from build123d import *

# Parameters (mm, degrees)
CROQUIS1_R              = 9.525
SALIENTE_EXTRUIR1_DEPTH = 10
CROQUIS2_R              = 9.525


with BuildPart() as part:
    # Croquis1 → Saliente-Extruir1 (new body)
    with BuildSketch(Plane(origin=(0, 0, 0), x_dir=(1, 0, 0), z_dir=(0, 1, 0))):
        with Locations(Location((0, 0, 0), (0, 0, 270))):
            Circle(CROQUIS1_R)
    extrude(amount=-SALIENTE_EXTRUIR1_DEPTH)

    # Barrer1: sweep along a curve in space
    with BuildLine() as barrer1_path:
        Line((0, -10, 0), (0, -50, 0))
        ThreePointArc((0, -50, 0), (4.393398282, -60.606601718, 0), (15, -65, 0))
        Line((15, -65, 0), (35, -65, 0))
        ThreePointArc((35, -65, 0), (45.606601718, -69.393398282, 0), (50, -80, 0))
        Line((50, -80, 0), (50, -145, 0))
        ThreePointArc((50, -145, 0), (54.393398282, -155.606601718, 0), (65, -160, 0))
        Line((65, -160, 0), (805, -160, 0))
        ThreePointArc((805, -160, 0), (815.606601718, -155.606601718, 0), (820, -145, 0))
        Line((820, -145, 0), (820, 175, 0))
        ThreePointArc((820, 175, 0), (820, 185.606601718, 4.393398282), (820, 190, 15))
        Line((820, 190, 15), (820, 190, 100))
    # Croquis2 → Barrer1 (sweep)
    with BuildSketch(Plane.XZ.offset(10)):
        Circle(CROQUIS2_R)
    sweep(path=barrer1_path.line)


solid = part.part
The listing builds one solid part. Answer for the finished solid, in the listing's coordinates (mm). A direction names the side the tool comes from. Give positions to 0.01 mm unless a question says otherwise; leave off trailing zeros. Loops run counter-clockwise (first coordinate to the right, second up) from the corner with the lowest first, then second, coordinate; pieces in that order, holes last. Notation, with made-up numbers: (-6.5, -23) - (7.5, -23) arc R19 ccw to (7.5, -15) - close; hole circle Ø8 at (72, 88). An arc over 180 degrees is marked (long way). Use one line per item in the form item = value.
1. Given pin 1 Ø9.5 at (x, z) = (-1, -2) entering from +Y, flat-ended and moving along its own axis, determine where the tip first touches the part or whether it passes through.
Calculated:
pin_1 = 0
2. Find the intervals of material crossed by line 1 along X through (y, z) = (184.5, 11); line 2 along Y through (x, z) = (338, 2), in increasing order. Write a range as [from, to].
Calculated:
line_1 = [811.71, 828.29]
line_2 = [-169.31, -150.69]
3. Section B-B on z = 69 is taken. Give the vertices of the cut face in (x, y) (3 decimals).
Calculated:
outline = circle Ø19.05 at (820, 190)
4. The mould has two halves that part along X. Classify faces 1 (the face through (440.18, -169.516, 0.419)), 2 (the face through (0, 0, 0)), 3 (the face through (821.24, 180.556, 58.095)): pulls with the +X half, pulls with the -X half, needs draft (parallel to the pull), parting line crosses it, or undercut.
Calculated:
face_1 = undercut
face_2 = needs draft
face_3 = parting line crosses it
5. Section A-A on x = 349 is taken. Give the vertices of the cut face in (y, z) (3 decimals).
Calculated:
outline = circle Ø19.05 at (-160, 0)
6. Which of the six approach directions +Z, -Z, +X, -X, +Y, -Y give full straight-line access (tool end or side, diameter ignored) to faces 4 (the face through (8.841, -25.35, 3.545)), 5 (the face through (820, 190, 100)), 6 (the face through (810.915, 17.24, 2.861))?
Calculated:
face_4 = +Y
face_5 = +Z, +X, -X, +Y, -Y
face_6 = none
